Geometry check sheet. Reference: the model listing, model coordinates, mm. Coordinates: 2 decimals unless noted, no trailing zeros. Write each loop counter-clockwise with the first axis right and the second up, starting at its lowest first coordinate (ties: lowest second). Pieces come first, ordered by that corner, then holes. Notation, with made-up numbers: (77, -24) -> (131, -24) arc R32 ccw to (131, 14) -> close; hole circle Ø5 at (67, 41.25). An arc over 180 degrees is marked (long way). One line per question, with ' | ' between items.
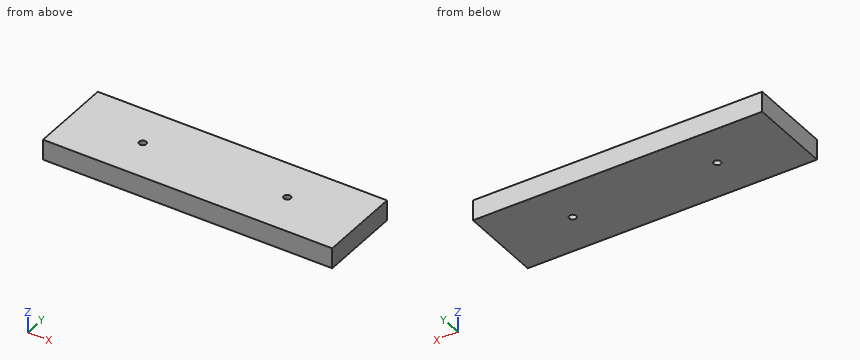
Autodesk Inventor part; units mm, degrees
ref_plane "YZ Plane" through (0, 0, 0) normal (1, 0, 0) x (0, 1, 0)
ref_plane "XZ Plane" through (0, 0, 0) normal (0, 1, 0) x (-1, 0, 0)
ref_plane "XY Plane" through (0, 0, 0) normal (0, 0, 1) x (1, 0, 0)
sketch "Sketch1" plane through (0, 0, 0) normal (0, 0, 1) x (1, 0, 0)
  line L0 (-67.6402, -19.558) -> (67.6402, -19.558)
  line L1 (67.6402, -19.558) -> (67.6402, 19.558)
  line L2 (67.6402, 19.558) -> (-67.6402, 19.558)
  line L3 (-67.6402, 19.558) -> (-67.6402, -19.558)
  line L4 (-67.6402, -19.558) -> (67.6402, 19.558) construction
  line L5 (67.6402, -19.558) -> (-67.6402, 19.558) construction
  point P0 (0, 0)
  dimension "d0" = 135.2804
  dimension "d1" = 39.116
extrude "Extrusion1" add sketch "Sketch1" along normal blind 9.525
sketch "Sketch2" plane through (0, 0, 9.525) normal (0, 0, 1) x (1, 0, 0)
  line L0 (-67.5894, 0) -> (67.7772, 0)
  line L1 (-67.6402, 19.558) -> (-67.6402, -19.558)
  line L2 (67.6402, -19.558) -> (67.6402, 19.558)
  line L3 (-67.6402, -19.558) -> (67.6402, -19.558)
  point P0 (0, 0)
  point P1 (-33.8074, 0)
  point P2 (33.8074, 0)
  dimension "d4" = 33.8328
  dimension "d5" = 33.8328
  dimension "d13" = 19.558
hole "Hole1" at (-33.8074, 0, 9.525) at (33.8074, 0, 9.525) direction (0, 0, -1) diameter 3.2512 end through all
properties part number "nmt_metalplate"
1. Material ranges on line 1 (X direction, y = 0, z = 6.5); line 2 (Y direction, x = 35, z = 5); line 3 (X direction, y = -1, z = 7), recorded low to high. Write a range as from..to.
Worked answers:
line 1: -67.64..-35.43, -32.18..32.18, 35.43..67.64 | line 2: -19.56..-1.1, 1.1..19.56 | line 3: -67.64..-35.09, -32.53..32.53, 35.09..67.64
2. Cross-section at A-A on y = 0. Record the boundary of the cut face in (x, z) (3 decimals).
Worked answers:
outline: (-67.64, 0) -> (-35.433, 0) -> (-35.433, 9.525) -> (-67.64, 9.525) -> close; (-32.182, 0) -> (32.182, 0) -> (32.182, 9.525) -> (-32.182, 9.525) -> close; (35.433, 0) -> (67.64, 0) -> (67.64, 9.525) -> (35.433, 9.525) -> close
3. Go/stop test with flat-tipped pins: P1, Ø10, axis at x = -14.5, y = -10.5, coming from the -Z side; P2, Ø2, axis at x = 33.81, y = 0, coming from the -Z side. Record where each tip stops, or that it passes through.
Worked answers:
P1: z = 0 | P2: through
